Geometry check sheet. Reference: the model listing, model coordinates, mm. A direction names the side the tool comes from. Give positions to 0.01 mm unless a question says otherwise; leave off trailing zeros. Loops run counter-clockwise (first coordinate to the right, second up) from the corner with the lowest first, then second, coordinate; pieces in that order, holes last. Notation, with made-up numbers: (74, 39) -> (97, 39) arc R30 ccw to (97, 66) -> close; hole circle Ø9 at (28, 2). An arc over 180 degrees is marked (long way). Write item = value, one per line.
```python
from build123d import *

# Parameters (mm, degrees)
BOSS_EXTRUDE1_DEPTH                 = 12.5
CUT_EXTRUDE1_REACH                  = 42.463
CUT_EXTRUDE1_END_RADIUS             = 9.5
CUT_EXTRUDE1_DIRECTION_2_REACH      = 42.463
CUT_EXTRUDE1_DIRECTION_2_END_RADIUS = 9.5
BOSS_EXTRUDE2_DEPTH                 = 6.35
SKETCH6_R                           = 2.5
BOSS_EXTRUDE3_DEPTH                 = 6.35
BOSS_EXTRUDE4_START                 = -46
BOSS_EXTRUDE4_DEPTH                 = 46
BOSS_EXTRUDE5_DEPTH                 = 6.35
BOSS_EXTRUDE5_DRAFT                 = 10
HOLE1_START                         = 6.15
HOLE1_OUTLINE_R                     = 2.5
HOLE1_DEPTH                         = 52.35
FILLET1_R                           = 2.5


# Read off the part's stored shape, not the designer's step: Hole1
with BuildPart() as part:
    # Sketch1 → Boss-Extrude1 (new, symmetric)
    with BuildSketch(Plane.XY):
        with BuildLine():
            ThreePointArc((-9.5, 12.87439319), (-35, 0), (-9.5, -12.87439319))
            ThreePointArc((-9.5, -12.87439319), (0, -9.748786379), (9.5, -12.87439319))
            ThreePointArc((9.5, -12.87439319), (35, 0), (9.5, 12.87439319))
            ThreePointArc((9.5, 12.87439319), (0, 9.748786379), (-9.5, 12.87439319))
        make_face()
    extrude(amount=BOSS_EXTRUDE1_DEPTH, both=True)

    # Sketch2 → Cut-Revolve1 (revolve, cut)
    with BuildSketch(Plane(origin=(19, 0, 0), x_dir=(0, 0, -1), z_dir=(1, 0, 0)), mode=Mode.PRIVATE) as cut_revolve1_sk:
        Polygon((-12.5, 0), (-12.5, 14.25), (-6.5, 14.25), (-6.5, 12.5), (-4.5, 12.5), (-4.5, 11.5), (-2.5, 11.5), (-2.5, 9.5), (9.5, 9.5), (9.5, 4.5), (8.5, 4.5), (8.5, 0), align=None)
    cut_revolve1 = revolve(cut_revolve1_sk.sketch.rotate(Axis((19, 0, -12.5), (0, 0, 1)), 90), axis=Axis((19, 0, -12.5), (0, 0, 1)), mode=Mode.SUBTRACT)

    # Mirror1: Cut-Revolve1 across plane
    add(cut_revolve1.mirror(Plane(origin=(0, 0, 0), x_dir=(0, 0, 1), z_dir=(1, 0, 0))), mode=Mode.SUBTRACT)

    # Cut-Extrude1: up to this cylinder (the profile starts outside it)
    cut_extrude1_end = Plane(origin=(19, 0, 0), z_dir=(0, 0, -1)) * Cylinder(CUT_EXTRUDE1_END_RADIUS, 104.926, mode=Mode.PRIVATE)
    # Sketch3 → Cut-Extrude1 (cut, up to the surface)
    with BuildSketch(Plane(origin=(0, 0, 0), x_dir=(0, 0, -1), z_dir=(1, 0, 0)), mode=Mode.PRIVATE) as cut_extrude1_sk1:
        with BuildLine():
            Line((-0.75, -7.75), (0.75, -7.75))
            ThreePointArc((0.75, -7.75), (1.810660172, -7.310660172), (2.25, -6.25))
            Line((2.25, -6.25), (2.25, 6.25))
            ThreePointArc((2.25, 6.25), (1.810660172, 7.310660172), (0.75, 7.75))
            Line((0.75, 7.75), (-0.75, 7.75))
            ThreePointArc((-0.75, 7.75), (-1.810660172, 7.310660172), (-2.25, 6.25))
            Line((-2.25, 6.25), (-2.25, -6.25))
            ThreePointArc((-2.25, -6.25), (-1.810660172, -7.310660172), (-0.75, -7.75))
        make_face()
    cut_extrude1_tool1 = extrude(cut_extrude1_sk1.sketch, amount=CUT_EXTRUDE1_REACH, mode=Mode.PRIVATE) - cut_extrude1_end
    add(cut_extrude1_tool1.solids().sort_by_distance((0, 0, 0))[0], mode=Mode.SUBTRACT)

    # Cut-Extrude1 direction 2: up to this cylinder (the profile starts outside it)
    cut_extrude1_direction_2_end = Plane(origin=(-19, 0, 0), z_dir=(0, 0, -1)) * Cylinder(CUT_EXTRUDE1_DIRECTION_2_END_RADIUS, 104.926, mode=Mode.PRIVATE)
    # Sketch3 → Cut-Extrude1 direction 2 (cut, up to the surface)
    with BuildSketch(Plane(origin=(0, 0, 0), x_dir=(0, 0, -1), z_dir=(1, 0, 0)), mode=Mode.PRIVATE) as cut_extrude1_direction_2_sk1:
        with BuildLine():
            Line((-0.75, -7.75), (0.75, -7.75))
            ThreePointArc((0.75, -7.75), (1.810660172, -7.310660172), (2.25, -6.25))
            Line((2.25, -6.25), (2.25, 6.25))
            ThreePointArc((2.25, 6.25), (1.810660172, 7.310660172), (0.75, 7.75))
            Line((0.75, 7.75), (-0.75, 7.75))
            ThreePointArc((-0.75, 7.75), (-1.810660172, 7.310660172), (-2.25, 6.25))
            Line((-2.25, 6.25), (-2.25, -6.25))
            ThreePointArc((-2.25, -6.25), (-1.810660172, -7.310660172), (-0.75, -7.75))
        make_face()
    cut_extrude1_direction_2_tool1 = extrude(cut_extrude1_direction_2_sk1.sketch, amount=-CUT_EXTRUDE1_DIRECTION_2_REACH, mode=Mode.PRIVATE) - cut_extrude1_direction_2_end
    add(cut_extrude1_direction_2_tool1.solids().sort_by_distance((0, 0, 0))[0], mode=Mode.SUBTRACT)

    # Sketch5 → Boss-Extrude2 (add)
    with BuildSketch(Plane.XY.offset(12.5)):
        with BuildLine():
            Line((-44.769952499, -5.044967379), (-34.999860317, -0.066856769))
            ThreePointArc((-34.999860317, -0.066856769), (-32.476862137, -8.624047016), (-25.763874629, -14.5))
            Line((-25.763874629, -14.5), (-42.5, -14.5))
            ThreePointArc((-42.5, -14.5), (-47.361849602, -10.667226819), (-44.769952499, -5.044967379))
        make_face()
    boss_extrude2 = extrude(amount=-BOSS_EXTRUDE2_DEPTH)

    # Mirror2: Boss-Extrude2 across plane
    add(boss_extrude2.mirror(Plane(origin=(0, 0, 0), x_dir=(0, 0, 1), z_dir=(1, 0, 0))))

    # Sketch6 → Boss-Extrude3 (add)
    with BuildSketch(Plane.XY.offset(12.5)):
        with BuildLine():
            Line((-24, 29.83), (-30.550716865, 11.071627699))
            ThreePointArc((-30.550716865, 11.071627699), (-20.3652292, 15.94164826), (-9.5, 12.87439319))
            ThreePointArc((-9.5, 12.87439319), (-8.605515622, 12.260083666), (-7.671449956, 11.707815773))
            Line((-7.671449956, 11.707815773), (-14, 29.83))
            ThreePointArc((-14, 29.83), (-19, 34.83), (-24, 29.83))
        make_face()
        with Locations((-19, 29.83)):
            Circle(SKETCH6_R, mode=Mode.SUBTRACT)
    extrude(amount=-BOSS_EXTRUDE3_DEPTH)

    # Sketch8 → Boss-Extrude4 (add)
    with BuildSketch(Plane(origin=(0, 0, 6.15), x_dir=(-1, 0, 0), z_dir=(0, 0, -1)).offset(BOSS_EXTRUDE4_START)):
        with BuildLine():
            Line((42.5, -14.5), (25.763874629, -14.5))
            ThreePointArc((25.763874629, -14.5), (17.40869711, -15.920670687), (9.5, -12.87439319))
            ThreePointArc((9.5, -12.87439319), (0, -9.748786379), (-9.5, -12.87439319))
            ThreePointArc((-9.5, -12.87439319), (-17.40869711, -15.920670687), (-25.763874629, -14.5))
            Line((-25.763874629, -14.5), (-42.5, -14.5))
            ThreePointArc((-42.5, -14.5), (0, -30.819495552), (42.5, -14.5))
        make_face()
    extrude(amount=BOSS_EXTRUDE4_DEPTH)


with BuildPart() as boss_extrude5_tool:
    # Sketch9 → Boss-Extrude5 (with draft: the straight prism first)
    with BuildSketch(Plane.XY.offset(52.15)):
        with BuildLine():
            Line((-7.5, 15.5), (-7.5, 9.15))
            ThreePointArc((-7.5, 9.15), (-19, -2.35), (-30.5, 9.15))
            Line((-30.5, 9.15), (-30.5, 15.5))
            Line((-30.5, 15.5), (-40, 15.5))
            Line((-40, 15.5), (-40, 7.918275005))
            ThreePointArc((-40, 7.918275005), (-41.230330983, 1.011790734), (-44.769952499, -5.044967379))
            ThreePointArc((-44.769952499, -5.044967379), (-47.361849602, -10.667226819), (-42.5, -14.5))
            ThreePointArc((-42.5, -14.5), (0, -30.819495552), (42.5, -14.5))
            ThreePointArc((42.5, -14.5), (47.361849602, -10.667226819), (44.769952499, -5.044967379))
            ThreePointArc((44.769952499, -5.044967379), (41.230330983, 1.011790734), (40, 7.918275005))
            Line((40, 7.918275005), (40, 15.5))
            Line((40, 15.5), (30.5, 15.5))
            Line((30.5, 15.5), (30.5, 9.15))
            ThreePointArc((30.5, 9.15), (19, -2.35), (7.5, 9.15))
            Line((7.5, 9.15), (7.5, 15.5))
            Line((7.5, 15.5), (-7.5, 15.5))
        make_face()
    extrude(amount=BOSS_EXTRUDE5_DEPTH)
    # Boss-Extrude5: the draft: its side faces are tilted about the plane it starts from
    boss_extrude5_sides = [boss_extrude5_tool.faces().sort_by_distance(p)[0] for p in [
        (41.230330983, 1.011790734, 55.325),
        (40, 11.709137503, 55.325),
        (35.25, 15.5, 55.325),
        (30.5, 12.325, 55.325),
        (19, -2.35, 55.325),
        (7.5, 12.325, 55.325),
        (0, 15.5, 55.325),
        (-7.5, 12.325, 55.325),
        (-19, -2.35, 55.325),
        (-30.5, 12.325, 55.325),
        (-35.25, 15.5, 55.325),
        (-40, 11.709137503, 55.325),
        (-41.230330983, 1.011790734, 55.325),
        (-47.361849602, -10.667226819, 55.325),
        (0, -30.819495552, 55.325),
        (47.361849602, -10.667226819, 55.325),
    ]]
    draft(boss_extrude5_sides, Plane.XY.offset(52.15), BOSS_EXTRUDE5_DRAFT)


with BuildPart() as part_1:
    add(part.part)

    # Boss-Extrude5: add boss_extrude5_tool
    add(boss_extrude5_tool.part)

    # Hole1 outline → Hole1 (cut)
    with BuildSketch(Plane.XY.offset(HOLE1_START)):
        with Locations((-42.5, -9.5)):
            Circle(HOLE1_OUTLINE_R)
    hole1 = extrude(amount=HOLE1_DEPTH, mode=Mode.SUBTRACT)

    # Mirror3: Hole1 across plane
    add(hole1.mirror(Plane(origin=(0, 0, 0), x_dir=(0, 0, 1), z_dir=(1, 0, 0))), mode=Mode.SUBTRACT)

    # Fillet1
    fillet1_edges = [part_1.edges().sort_by_distance(p)[0] for p in [
        (35, 0, -12.5),
        (0, -9.748786379, -12.5),
        (-35, 0, -12.5),
        (0, 9.748786379, -12.5),
    ]]
    fillet(fillet1_edges, radius=FILLET1_R)


solid = part_1.part
```
Item 1: Gauge pin test, flat ends, axial feed: pin 1 (4 mm diameter, centred on x = 22, y = 14, fed in from +Z); pin 2 (6 mm diameter, centred on x = -19, y = 5, fed in from +Z); pin 3 (10 mm diameter, centred on x = 10, z = 27, fed in from +Y). Record the tip position at first contact, or that the pin passes through.
Answer:
pin_1 = 12.5
pin_2 = -8.5
pin_3 = -10.55
Item 2: Tool access check on faces 1 (the flat face through (-4, 2, 12.5)), 2 (the cylindrical face through (8.03, -3.45, 3.49)), 3 (the flat face through (-31.05, 12.28, 55.28)), 4 (the flat face through (-39.95, -2.59, 9.37)). Record the directions out of +Z, -Z, +X, -X, +Y, -Y that give a thin tool (end or side, any length) a straight path to the whole face; none if there is none.
Answer:
face_1 = +Y
face_2 = none
face_3 = +Z, +Y
face_4 = -Z, -X, +Y
Item 3: Thickness scan on L1, parallel to Y at x = 19, z = -6; L2, parallel to Z at x = -39.5, y = -5; L3, parallel to X at y = -1.5, z = 6. Record the ranges inside material, lowest first. Write a range as [from, to].
Answer:
L1 = [-16, -9.5], [9.5, 16]
L2 = [6.15, 12.5], [52.15, 58.5]
L3 = [-34.93, -31.41], [-6.59, 6.59], [31.41, 34.93]
Item 4: Section check A-A, the plane z = 40.5. Record the cut outline in (x, y), plus the area to 4 significant figures.
Answer:
outline = (-42.5, -14.5) arc R63.5 ccw to (42.5, -14.5) -> (25.76, -14.5) arc R16 cw to (9.5, -12.87) arc R16 ccw to (-9.5, -12.87) arc R16 cw to (-25.76, -14.5) -> close
area = 1,000 mm^2
Item 5: Draft check along Z on faces 5 (the flat face through (-1, -12, 58.5)), 6 (the flat face through (39.95, -2.59, 9.37)), 7 (the flat face through (8, 4, 4.5)), 8 (the flat face through (0, 0, 2.25)). Enter one of: +Z half, -Z half, draft (parallel to the pull), parting line (faces both ways), or undercut.
Answer:
face_5 = +Z half
face_6 = draft
face_7 = undercut
face_8 = undercut
